```python
from build123d import *

# Parameters (mm, degrees)
F1_DEPTH = 16
F2_DEPTH = 7
F3_DEPTH = 4
F4_R     = 2
F5_R     = 1.9999
F6_R     = 3
F7_SIZE  = 0.5


# Not quite as in the source:
# - a fillet or chamfer is up to 0.001 mm smaller than in the source, because OpenCascade refuses the exact size
# - a feature names something its author has since deleted; it is built from what else it names


with BuildPart() as f1:
    # F0 (on Front) → F1 (new body)
    with BuildSketch(Plane.XZ):
        with BuildLine():
            ThreePointArc((-5.7041860158, 8.815455853), (0, 10.5), (5.7041860158, 8.815455853))
            Line((5.7041860158, 8.815455853), (7.2831998462, 10.3944696834))
            Line((7.2831998462, 10.3944696834), (0, 17.6776695297))
            Line((0, 17.6776695297), (-7.2831998462, 10.3944696834))
            Line((-7.2831998462, 10.3944696834), (-5.7041860158, 8.815455853))
        make_face()
        with BuildLine():
            ThreePointArc((-8.815455853, 5.7041860158), (-7.4246212025, 7.4246212025), (-5.7041860158, 8.815455853))
            Line((-5.7041860158, 8.815455853), (-7.2831998462, 10.3944696834))
            Line((-7.2831998462, 10.3944696834), (-10.3944696834, 7.2831998462))
            Line((-10.3944696834, 7.2831998462), (-8.815455853, 5.7041860158))
        make_face()
        with BuildLine():
            ThreePointArc((-8.815455853, -5.7041860158), (-10.5, 0), (-8.815455853, 5.7041860158))
            Line((-8.815455853, 5.7041860158), (-10.3944696834, 7.2831998462))
            Line((-10.3944696834, 7.2831998462), (-17.6776695297, 0))
            Line((-17.6776695297, 0), (-10.3944696834, -7.2831998462))
            Line((-10.3944696834, -7.2831998462), (-8.815455853, -5.7041860158))
        make_face()
        with BuildLine():
            ThreePointArc((5.7041860158, 8.815455853), (7.4246212025, 7.4246212025), (8.815455853, 5.7041860158))
            Line((8.815455853, 5.7041860158), (10.3944696834, 7.2831998462))
            Line((10.3944696834, 7.2831998462), (7.2831998462, 10.3944696834))
            Line((7.2831998462, 10.3944696834), (5.7041860158, 8.815455853))
        make_face()
        Polygon((0, 17.6776695297), (7.2831998462, 10.3944696834), (10.111626971, 13.2228968082), (0, 23.3345237792), (-10.111626971, 13.2228968082), (-7.2831998462, 10.3944696834), align=None)
        Polygon((7.2831998462, 10.3944696834), (10.3944696834, 7.2831998462), (13.2228968082, 10.111626971), (10.111626971, 13.2228968082), align=None)
        Polygon((-10.3944696834, 7.2831998462), (-7.2831998462, 10.3944696834), (-10.111626971, 13.2228968082), (-13.2228968082, 10.111626971), align=None)
        Polygon((-17.6776695297, 0), (-10.3944696834, 7.2831998462), (-13.2228968082, 10.111626971), (-20.5060966544, 2.8284271247), (-26, 8.3223304703), (-26, 2.6654762208), (-13.2228968082, -10.111626971), (-10.3944696834, -7.2831998462), align=None)
        Polygon((-13.2228968082, 10.111626971), (-10.111626971, 13.2228968082), (-12.9400540957, 16.0513239329), (-16.0513239329, 12.9400540957), align=None)
        Polygon((17.6776695297, 0), (10.3944696834, -7.2831998462), (13.2228968082, -10.111626971), (26, 2.6654762208), (26, 8.3223304703), (20.5060966544, 2.8284271247), (13.2228968082, 10.111626971), (10.3944696834, 7.2831998462), align=None)
        with BuildLine():
            ThreePointArc((8.815455853, 5.7041860158), (10.5, 0), (8.815455853, -5.7041860158))
            Line((8.815455853, -5.7041860158), (10.3944696834, -7.2831998462))
            Line((10.3944696834, -7.2831998462), (17.6776695297, 0))
            Line((17.6776695297, 0), (10.3944696834, 7.2831998462))
            Line((10.3944696834, 7.2831998462), (8.815455853, 5.7041860158))
        make_face()
        Polygon((16.0513239329, 12.9400540957), (13.2228968082, 10.111626971), (20.5060966544, 2.8284271247), (26, 8.3223304703), (26, 12), (20, 12), (20, 32), (0, 32), (-20, 32), (-20, 12), (-26, 12), (-26, 8.3223304703), (-20.5060966544, 2.8284271247), (-13.2228968082, 10.111626971), (-16.0513239329, 12.9400540957), (-12.9400540957, 16.0513239329), (-10.111626971, 13.2228968082), (0, 23.3345237792), (10.111626971, 13.2228968082), (12.9400540957, 16.0513239329), align=None)
        Polygon((10.111626971, 13.2228968082), (13.2228968082, 10.111626971), (16.0513239329, 12.9400540957), (12.9400540957, 16.0513239329), align=None)
        Polygon((26, 2.6654762208), (13.2228968082, -10.111626971), (17.4655374953, -14.3542676581), (26, -5.8198051534), align=None)
        Polygon((-16.0513239329, -12.9400540957), (-13.2228968082, -10.111626971), (-26, 2.6654762208), (-26, -2.9913780286), align=None)
    extrude(amount=-F1_DEPTH)

    # F0 (on Front) → F2 (cut)
    with BuildSketch(Plane.XZ):
        Polygon((10.111626971, 13.2228968082), (13.2228968082, 10.111626971), (16.0513239329, 12.9400540957), (12.9400540957, 16.0513239329), align=None)
        Polygon((7.2831998462, 10.3944696834), (10.3944696834, 7.2831998462), (13.2228968082, 10.111626971), (10.111626971, 13.2228968082), align=None)
        with BuildLine():
            ThreePointArc((5.7041860158, 8.815455853), (7.4246212025, 7.4246212025), (8.815455853, 5.7041860158))
            Line((8.815455853, 5.7041860158), (10.3944696834, 7.2831998462))
            Line((10.3944696834, 7.2831998462), (7.2831998462, 10.3944696834))
            Line((7.2831998462, 10.3944696834), (5.7041860158, 8.815455853))
        make_face()
        with BuildLine():
            ThreePointArc((-8.815455853, 5.7041860158), (-7.4246212025, 7.4246212025), (-5.7041860158, 8.815455853))
            Line((-5.7041860158, 8.815455853), (-7.2831998462, 10.3944696834))
            Line((-7.2831998462, 10.3944696834), (-10.3944696834, 7.2831998462))
            Line((-10.3944696834, 7.2831998462), (-8.815455853, 5.7041860158))
        make_face()
        Polygon((-13.2228968082, 10.111626971), (-10.111626971, 13.2228968082), (-12.9400540957, 16.0513239329), (-16.0513239329, 12.9400540957), align=None)
        Polygon((-10.3944696834, 7.2831998462), (-7.2831998462, 10.3944696834), (-10.111626971, 13.2228968082), (-13.2228968082, 10.111626971), align=None)
    extrude(amount=-F2_DEPTH, mode=Mode.SUBTRACT)

    # F0 (on Front) → F3 (cut)
    with BuildSketch(Plane.XZ):
        Polygon((0, 17.6776695297), (7.2831998462, 10.3944696834), (10.111626971, 13.2228968082), (0, 23.3345237792), (-10.111626971, 13.2228968082), (-7.2831998462, 10.3944696834), align=None)
        Polygon((17.6776695297, 0), (10.3944696834, -7.2831998462), (13.2228968082, -10.111626971), (26, 2.6654762208), (26, 8.3223304703), (20.5060966544, 2.8284271247), (13.2228968082, 10.111626971), (10.3944696834, 7.2831998462), align=None)
        Polygon((-17.6776695297, 0), (-10.3944696834, 7.2831998462), (-13.2228968082, 10.111626971), (-20.5060966544, 2.8284271247), (-26, 8.3223304703), (-26, 2.6654762208), (-13.2228968082, -10.111626971), (-10.3944696834, -7.2831998462), align=None)
    extrude(amount=-F3_DEPTH, mode=Mode.SUBTRACT)

    # F4
    f4_edges = [f1.edges().sort_by_distance(p)[0] for p in [
        (-16.051324, 3.5, 12.940054),
        (-12.940054, 3.5, 16.051324),
        (12.940054, 3.5, 16.051324),
        (16.051324, 3.5, 12.940054),
        (0, 2, 23.334524),
    ]]
    fillet(f4_edges, radius=F4_R)

    # F5 (radius 2 in the source; OpenCascade refuses exactly that, so slightly less here)
    f5_edges = [f1.edges().sort_by_distance(p)[0] for p in [
        (19.611448, 4, -3.723075),
        (14.03607, 4, -3.6416),
        (14.03607, 4, 3.6416),
        (16.864497, 4, 6.470027),
        (5.76292, 4, 17.571604),
        (-16.864497, 4, 6.470027),
        (-23.253048, 4, 5.575379),
        (-14.03607, 4, -3.6416),
        (-3.6416, 4, 14.03607),
        (-14.03607, 4, 3.6416),
        (-19.611448, 4, -3.723075),
        (23.253048, 4, 5.575379),
        (0, 4, 22.506097),
        (-5.76292, 4, 17.571604),
        (3.6416, 4, 14.03607),
    ]]
    fillet(f5_edges, radius=F5_R)

    # F6
    f6_edges = [f1.edges().sort_by_distance(p)[0] for p in [
        (17.465537, 8, -14.354268),
        (-16.051324, 8, -12.940054),
        (26, 8, -5.819805),
        (-26, 8, -2.991378),
    ]]
    fillet(f6_edges, radius=F6_R)

    # F7
    f7_edges = [f1.edges().sort_by_distance(p)[0] for p in [
        (20, 8, 32),
        (26, 8, 12),
        (-20, 8, 32),
        (-26, 8, 12),
    ]]
    chamfer(f7_edges, length=F7_SIZE)


solid = f1.part
```
Check sheet for the modelled part. Datum: model origin and axes. Units: mm. A direction names the side the tool comes from. Coordinates: 2 decimals unless noted, no trailing zeros. Write each loop counter-clockwise with the first axis right and the second up, starting at its lowest first coordinate (ties: lowest second). Pieces come first, ordered by that corner, then holes. Notation, with made-up numbers: M 85,85 L 89,85 A25 cw 89,122 Z; hole C 66,57.25 d11. An arc over 180 degrees is marked long. Write item = value, one per line. Start each with the question number.
1. Thickness scan on probe 1 along X at (y, z) = (5, 0); probe 2 along X at (y, z) = (1.25, 0.5); probe 3 along X at (y, z) = (5.5, 7). Record the ranges inside material, lowest first.
2. Tool access check on faces 5 (the cylindrical face through (-15.11, 3.43, 3.42)), 6 (the flat face through (12, 0, 0)), 7 (the flat face through (23.29, 0.99, 5.61)). Record the directions out of +Z, -Z, +X, -X, +Y, -Y that give a thin tool (end or side, any length) a straight path to the whole face; none if there is none.
3. Mould release check, pull along Z, two halves, no side actions. Record for faces 1 (the cylindrical face through (25.78, 8.11, -5.71)), 2 (the flat face through (0, 0, 24)), 3 (the cylindrical face through (-3.3, 3.43, 15.23)), 4 (the flat face through (11, 7, 11)): pulls with the +Z half, pulls with the -Z half, needs draft (parallel to the pull), parting line crosses it, or undercut.
4. Sectioned sample at B-B (z = 27.5). Record the cut outline in (x, y), then the cut area to 3 significant figures.
5. Go/stop test with flat-tipped pins: pin 1 (1 mm diameter, centred on x = 15, z = -6, fed in from -Y); pin 2 (1.5 mm diameter, centred on x = -20, z = -1, fed in from -Y). Record where each tip stops, or that it passes through.
6. Sectioned sample at C-C (y = 12). Record the cut outline in (x, z).
The answers:
q1.probe_1 = -26 to -10.5, 10.5 to 26
q1.probe_2 = -26 to -23.83, -17.18 to -10.49, 10.49 to 17.18, 23.83 to 26
q1.probe_3 = -26 to -10.11, 10.11 to 26
q2.face_5 = -Y
q2.face_6 = +Z, -Z, +X, -X, -Y
q2.face_7 = +X, -Y
q3.face_1 = pulls with the -Z half
q3.face_2 = needs draft
q3.face_3 = undercut
q3.face_4 = undercut
q4.outline = M -20,0 L 20,0 L 20,16 L -20,16 Z
q4.area = 640 mm²
q5.pin_1 = 3.81
q5.pin_2 = 3.67
q6.outline = M -26,-1.75 A3 ccw -25.12,-3.87 L -18.17,-10.82 A3 ccw -13.93,-10.82 L -8.82,-5.7 A10.5 cw long 8.82,-5.7 L 15.34,-12.23 A3 ccw 19.59,-12.23 L 25.12,-6.7 A3 ccw 26,-4.58 L 26,11.5 L 25.5,12 L 20,12 L 20,31.5 L 19.5,32 L -19.5,32 L -20,31.5 L -20,12 L -25.5,12 L -26,11.5 Z
